from build123d import *

# Parameters (mm, degrees)
F0_W     = 132.1267485619
F0_H     = 88.8679325581
F1_DEPTH = 41.7771711946
F2_SIZE  = 12.7
F3_R     = 21.6691340714
F4_DEPTH = 276.723921299
F5_SIZE  = 5.08
F6_R     = 4.579207341
F7_DEPTH = 88.8689325581
F6_R_2   = 4.4293082264
F8_DEPTH = 88.8689325581
F9_T     = -2.54


with BuildPart() as f1:
    # F0 (on Front) → F1 (new body)
    with BuildSketch(Plane.XZ):
        Rectangle(F0_W, F0_H)
    extrude(amount=F1_DEPTH)

    # F2
    f2_edges = [f1.edges().sort_by_distance(p)[0] for p in [
        (0, -41.777171, -44.433966),
        (66.063374, -41.777171, 0),
        (0, -41.777171, 44.433966),
        (-66.063374, -41.777171, 0),
        (0, 0, -44.433966),
        (66.063374, 0, 0),
        (-66.063374, 0, 0),
        (0, 0, 44.433966),
    ]]
    chamfer(f2_edges, length=F2_SIZE)

    # F3 (on face) → F4 (cut)
    with BuildSketch(Plane.XZ.offset(41.7771711946)):
        Circle(F3_R)
    extrude(amount=-F4_DEPTH, mode=Mode.SUBTRACT)

    # F5
    f5_edges = [f1.edges().sort_by_distance(p)[0] for p in [
        (-21.669134, 0, 0),
        (-21.669134, -41.777171, 0),
    ]]
    chamfer(f5_edges, length=F5_SIZE)

    # F6 (on face) → F7 (cut, through all)
    with BuildSketch(Plane.XY.offset(44.433966279)):
        with Locations((-43.1207939982, -20.8885855973)):
            Circle(F6_R)
    extrude(amount=-F7_DEPTH, mode=Mode.SUBTRACT)

    # F6 (on face) → F8 (cut, through all)
    with BuildSketch(Plane.XY.offset(44.433966279)):
        with Locations((-43.1207939982, -20.8885855973)):
            Circle(F6_R)
        with Locations((51.215508439, -20.8885855973)):
            Circle(F6_R_2)
    extrude(amount=-F8_DEPTH, mode=Mode.SUBTRACT)

    # F9
    f9_openings = [f1.faces().sort_by_distance(p)[0] for p in [
        (-27.990858, 0, 0),
    ]]
    offset(amount=F9_T, openings=f9_openings)


solid = f1.part
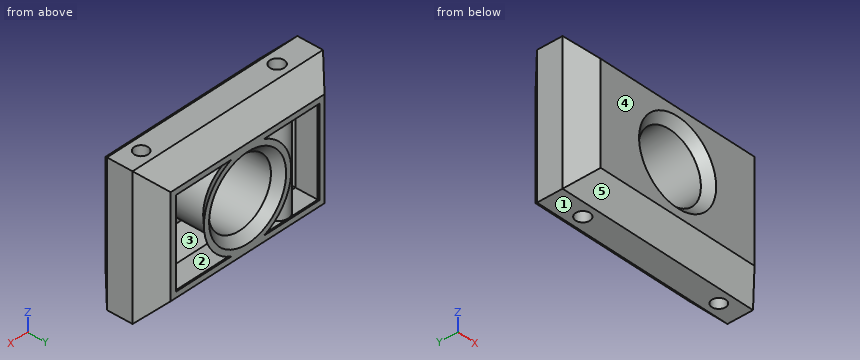
For this review, take the finished solid that the model builds, in its own axes (mm). Face numbers are marked on the shaded views. A direction names the side the tool comes from. Give positions to 0.01 mm unless a question says otherwise; leave off trailing zeros. Order: outer loops, then holes, each group sorted by start corner. A loop starts at its lowest first (then second) coordinate and runs counter-clockwise, first axis right, second up. Notation, with made-up numbers: M 66.5,28.5 L 109.5,28.5 A28 ccw 109.5,49.5 Z; hole C 28.25,23 d10. An arc over 180 degrees is marked long. Answer in a Markdown table with one row per item. Add a question column.
(1) Consider section A-A on z = -38. State the section outline as (x, y) points, and give its area (3 significant figures).
(2) For pin 1 (12 mm diameter, centred on x = -11, y = -6, fed in from -Z), flat-tipped, find the tip position at first contact; note if it passes through.
(3) Consider section D-D on x = 0. Give the number of separate pieces and of enclosed holes in the cut face, and give its area (3 significant figures).
(4) Consider section C-C on y = -11. State the section outline as (x, z) points.
(5) Consider section B-B on x = -40. State the section outline as (y, z) points, and give its area (3 significant figures).
(6) For the marked faces 1 and 2, list the 3-axis set-ups (+Z, -Z, +X, -X, +Y, -Y) from which the entire face can be reached by the end or side of a thin tool; tool diameter is ignored.
(7) Wall thickness on probe 1 along Z at (x, y) = (0, -27); probe 2 along X at (y, z) = (-15, -19); probe 3 along Z at (x, y) = (1.5, -31.5): over which ranges is each line inside the solid? List them lowest first. Write a range as [from, to].
(8) Mouldability with a two-part tool opening along Z and no side actions: class the marked faces 3, 4 and 5 as +Z half, -Z half, draft (parallel to the pull), parting line (faces both ways), or undercut.
Evaluation:
| question | item | result |
|---|---|---|
| 1 | outline | M -66.06,-29.08 L -59.63,-35.51 L 59.63,-35.51 L 66.06,-29.08 L 66.06,-12.7 L 59.63,-6.27 L -59.63,-6.27 L -66.06,-12.7 Z; C -43.12,-20.89 d14.24; C 51.22,-20.89 d13.94; hole M -63.52,-28.03 L -59.63,-31.92 L 59.63,-31.92 L 63.52,-28.03 L 63.52,-13.75 L 59.63,-9.86 L -59.63,-9.86 L -63.52,-13.75 Z; hole C -43.12,-20.89 d9.16; hole C 51.22,-20.89 d8.86 |
| 1 | area | 1,190 mm^2 |
| 2 | pin 1 | stops at z = -43.73 |
| 3 | separate pieces | 2 |
| 3 | enclosed holes | 2 |
| 3 | area | 503 mm^2 |
| 4 | outline | M -64.36,-42.73 L 64.36,-42.73 L 64.36,42.73 L -64.36,42.73 Z; C 0,0 d48.42; hole M -60.77,-39.14 L 60.77,-39.14 L 60.77,39.14 L -60.77,39.14 Z; hole C 0,0 d43.34 |
| 5 | outline | M -41.78,-31.73 L -29.08,-44.43 L -24.24,-44.43 L -24.24,44.43 L -29.08,44.43 L -41.78,31.73 Z; M -17.54,-44.43 L -12.7,-44.43 L 0,-31.73 L 0,-28.14 L -13.75,-41.89 L -14.49,-41.89 L -14.49,41.89 L -13.75,41.89 L 0,28.14 L 0,31.73 L -12.7,44.43 L -17.54,44.43 Z; hole M -39.24,-30.68 L -28.03,-41.89 L -27.29,-41.89 L -27.29,41.89 L -28.03,41.89 L -39.24,30.68 Z |
| 5 | area | 894 mm^2 |
| 6 | face 1 | -Z, +X, -X, +Y, -Y |
| 6 | face 2 | none |
| 7 | probe 1 | z = [-44.43, -41.89], [-24.21, -21.67], [21.67, 24.21], [41.89, 44.43] |
| 7 | probe 2 | x = [-66.06, -63.52], [-47.12, -39.12], [-15, -10.42], [10.42, 15], [47.49, 54.94], [63.52, 66.06] |
| 7 | probe 3 | z = [-42.01, -38.42], [-24.16, -21.62], [21.62, 24.16], [38.42, 42.01] |
| 8 | face 3 | undercut |
| 8 | face 4 | draft |
| 8 | face 5 | -Z half |
